Build history of the part. All positions in model axes, mm. Face numbers are marked on the shaded views. Give positions to 0.01 mm unless a question says otherwise; leave off trailing zeros. Order: outer loops, then holes, each group sorted by start corner. A loop starts at its lowest first (then second) coordinate and runs counter-clockwise, first axis right, second up. Notation, with made-up numbers: (67.25, 16.5) - (102.25, 16.5) arc R20 ccw to (102.25, 46.5) - close; hole circle Ø10 at (-21.75, 43.5). An arc over 180 degrees is marked (long way). Use a Markdown table: item, result.
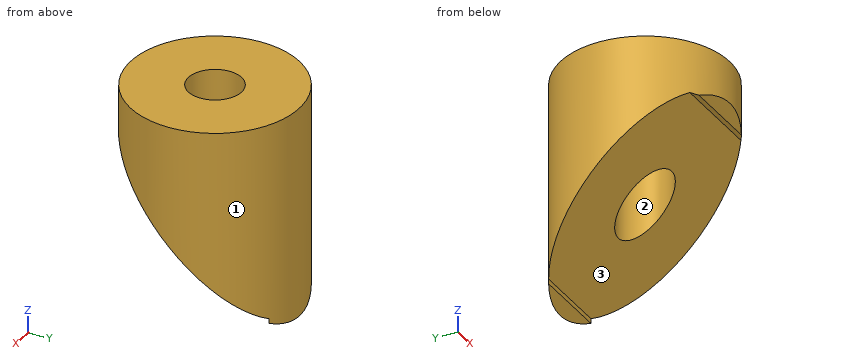
from build123d import *

# Parameters (mm, degrees)
BOSS_EXTRUDE1_DEPTH     = 9.525
SKETCH2_OUTSIDE_W       = 27.65
SKETCH2_OUTSIDE_H       = 27.65
SKETCH2_OUTSIDE_R       = 6.35
CUT_EXTRUDE1_DEPTH      = 20.05
CUT_EXTRUDE1_DEPTH_BACK = 1
SKETCH3_R               = 2
CUT_EXTRUDE2_DEPTH      = 16.875
CUT_EXTRUDE6_DEPTH      = 7.35
CUT_EXTRUDE6_DEPTH_BACK = 7.35


with BuildPart() as part:
    # Sketch1 → Boss-Extrude1 (new body, symmetric)
    with BuildSketch(Plane(origin=(0, 0, 0), x_dir=(0, 0, -1), z_dir=(1, 0, 0))):
        Polygon((19.05, 9.525), (0, -9.525), (0, 9.525), align=None)
    extrude(amount=BOSS_EXTRUDE1_DEPTH, both=True)

    # Sketch2 outside → Cut-Extrude1 (cut, two sides)
    with BuildSketch(Plane(origin=(0, -2.789807909, 0), x_dir=(1, 0, 0), z_dir=(0, 0, -1))) as cut_extrude1_sk:
        with Locations((0, -2.79)):
            Rectangle(SKETCH2_OUTSIDE_W, SKETCH2_OUTSIDE_H)
        with Locations((0, -2.789807909)):
            Circle(SKETCH2_OUTSIDE_R, mode=Mode.SUBTRACT)
    extrude(amount=CUT_EXTRUDE1_DEPTH, mode=Mode.SUBTRACT)
    extrude(cut_extrude1_sk.sketch, amount=-CUT_EXTRUDE1_DEPTH_BACK, mode=Mode.SUBTRACT)

    # Sketch3 → Cut-Extrude2 (cut, through all)
    with BuildSketch(Plane.XY):
        Circle(SKETCH3_R)
    extrude(amount=-CUT_EXTRUDE2_DEPTH, mode=Mode.SUBTRACT)

    # Sketch11 → Cut-Extrude6 (cut, two sides)
    with BuildSketch(Plane(origin=(0, 0, 0), x_dir=(0, 0, -1), z_dir=(1, 0, 0))) as cut_extrude6_sk:
        Polygon((15.15657951, 5.63157951), (14.797369265, 5.63157951), (3.89342049, -5.272369265), (3.89342049, -5.63157951), align=None)
    extrude(amount=CUT_EXTRUDE6_DEPTH, mode=Mode.SUBTRACT)
    extrude(cut_extrude6_sk.sketch, amount=-CUT_EXTRUDE6_DEPTH_BACK, mode=Mode.SUBTRACT)


solid = part.part
1) Pin check, flat tips, straight feed: P1, Ø1, axis at x = 4.5, z = -10.5, coming from the +Y side; P2, Ø2.5, axis at x = 0, y = 0, coming from the +Z side; P3, Ø4, axis at x = 5, z = -7, coming from the +Y side; P4, Ø5, axis at x = -1, y = 2, coming from the -Z side. Stop position of each tip, or through.
Computed:
| item | result |
|---|---|
| P1 | stops at y = 4.93 |
| P2 | passes through |
| P3 | stops at y = 5.6 |
| P4 | stops at z = -13.67 |
2) Slice it at D-D (x = 3.25). Write the cut outline in (y, z).
Computed:
| item | result |
|---|---|
| outline | (-5.46, -3.89) - (-5.27, -3.89) - (5.46, -14.62) - (5.46, 0) - (-5.46, 0) - close |
3) Slice it at C-C (z = -5). Write the cut outline in (x, y).
Computed:
| item | result |
|---|---|
| outline | (-4.79, -4.17) - (4.79, -4.17) arc R6.35 ccw (long way) to start; hole circle Ø4 at (0, 0) |
4) Slice it at B-B (x = 0). Write the cut outline in (y, z) (3 decimals), and give its area (3 significant figures).
Computed:
| item | result |
|---|---|
| outline | (-6.35, -3.175) - (-5.632, -3.893) - (-5.272, -3.893) - (-2, -7.166) - (-2, 0) - (-6.35, 0) - close; (2, -11.166) - (5.632, -14.797) - (5.632, -15.157) - (6.35, -15.875) - (6.35, 0) - (2, 0) - close |
| area | 80.3 mm² |
5) Slice it at A-A (y = -0.25). Write the cut outline in (x, z), and give its area (3 significant figures).
Computed:
| item | result |
|---|---|
| outline | (-6.35, -8.92) - (-1.98, -8.92) - (-1.98, 0) - (-6.35, 0) - close; (1.98, -8.92) - (6.35, -8.92) - (6.35, 0) - (1.98, 0) - close |
| area | 77.8 mm² |
6) Two-plate mould, pull along Y, no slides. Class the marked faces 1, 2 and 3: +Y half, -Y half, draft (parallel to the pull), parting line (faces both ways), or undercut.
Computed:
| item | result |
|---|---|
| face 1 | parting line |
| face 2 | undercut |
| face 3 | -Y half |
7) Wall check: line 1 (Y direction, x = 0, z = -2.5); line 2 (Y direction, x = 0, z = -8.5). Give the ranges that are in metal, low to high. Write a range as from..to.
Computed:
| item | result |
|---|---|
| line 1 | y = -6.35..-2, 2..6.35 |
| line 2 | y = 2..6.35 |
